Here's how the part is built. I have some questions about the finished solid (model axes, mm). A direction names the side the tool comes from. Round coordinates to 2 decimals unless told otherwise and drop trailing zeros. Order: outer loops, then holes, each group sorted by start corner. A loop starts at its lowest first (then second) coordinate and runs counter-clockwise, first axis right, second up.
```python
from build123d import *

# Parameters (mm, degrees)
RADYUS1_R             = 10
IZIM2_R               = 3.75
KES_EKSTR_ZYON1_DEPTH = 10
RADYUS2_R             = 10
IZIM3_R               = 3.5
KES_EKSTR_ZYON2_DEPTH = 100.511524539


with BuildPart() as part:
    # Çizim1 → Döndür1 (revolve)
    with BuildSketch(Plane.XY):
        Polygon((158.555065461, 64.488475461), (158.555065461, 62.488475461), (48.555065461, 62.488475461), (48.555065461, 23.488475461), (888.555065461, 23.488475461), (888.555065461, 62.488475461), (778.555065461, 62.488475461), (778.555065461, 64.488475461), (688.555065461, 64.488475461), (688.555065461, 83.488475461), (248.555065461, 83.488475461), (248.555065461, 64.488475461), align=None)
    revolve(axis=Axis((48.555065461, 23.488475461, 0), (1, 0, 0)))

    # Radyus1
    radyus1_edges = [part.edges().sort_by_distance(p)[0] for p in [
        (48.555065461, -15.511524539, 0),
    ]]
    fillet(radyus1_edges, radius=RADYUS1_R)

    # Çizim2 → Kes-Ekstrüzyon1 (cut)
    with BuildSketch(Plane.ZY.offset(-48.555065461)):
        with Locations((0, 23.488475461)):
            Circle(IZIM2_R)
    extrude(amount=-KES_EKSTR_ZYON1_DEPTH, mode=Mode.SUBTRACT)

    # Radyus2
    radyus2_edges = [part.edges().sort_by_distance(p)[0] for p in [
        (888.555065461, -15.511524539, 0),
    ]]
    fillet(radyus2_edges, radius=RADYUS2_R)

    # Çizim3 → Kes-Ekstrüzyon2 (cut, through all)
    with BuildSketch(Plane(origin=(0, 63, 0), x_dir=(1, 0, 0), z_dir=(0, 1, 0))):
        with Locations((63.555065461, 0)):
            Circle(IZIM3_R)
        with Locations((873.555065461, 0)):
            Circle(IZIM3_R)
    extrude(amount=-KES_EKSTR_ZYON2_DEPTH, mode=Mode.SUBTRACT)


solid = part.part
```
1) I'm going to push flat-ended pins straight in: pin 1 (3 mm diameter, centred on x = 761.5, z = -6.5, fed in from -Y); pin 2 (10 mm diameter, centred on y = 52.5, z = 36.5, fed in from -X); pin 3 (10 mm diameter, centred on x = 472.5, y = 26, fed in from -Z); pin 4 (6.5 mm diameter, centred on x = 873.56, z = 0, fed in from +Y). Where does each tip first touch, or does it pass through?
2) If we section it at A-A (x = 364): Write out the boundary of the cut face in (y, z), plus the area to 3 significant figures.
3) If we section it at D-D (x = 120): Write out the boundary of the cut face in (y, z), plus the area to 3 significant figures.
4) If we section it at B-B (y = 8.5): Give the number of separate pieces and of enclosed holes in the cut face, plus the area to 3 significant figures.
5) For faces 1 (the cylindrical face through (465.475, -36.454, 2.638)), 2 (the cylindrical face through (107.86, 60.69, 11.71)), 3 (the flat face through (688.555, -16, -12)), which set-ups out of +Z, -Z, +X, -X, +Y, -Y let a thin tool reach every point of the face, with its end or its side?
6) If we section it at C-C (y = 74): Write out the boundary of the cut face in (x, z), plus the area to 3 significant figures.
7) I need wall thicknesses on line 1 (X direction, y = 17, z = 0); line 2 (X direction, y = 24.5, z = 0); line 3 (X direction, y = 43.5, z = -53). Which ranges of each line are inside material? Lowest first, please.
Solutions:
1. pin 1: stops at y = -17.21
1. pin 2: stops at x = 248.56
1. pin 3: stops at z = -60
1. pin 4: passes through
2. outline: circle Ø120 at (23.49, 0)
2. area: 11,300 mm2
3. outline: circle Ø78 at (23.49, 0)
3. area: 4,780 mm2
4. separate pieces: 1
4. enclosed holes: 2
4. area: 80,500 mm2
5. face 1: +X, -X
5. face 2: -X
5. face 3: +X
6. outline: (248.56, -32.38) - (688.56, -32.38) - (688.56, 32.38) - (248.56, 32.38) - close
6. area: 28,500 mm2
7. line 1: x = 48.56 to 60.06, 67.06 to 870.06, 877.06 to 888.56
7. line 2: x = 58.56 to 60.06, 67.06 to 870.06, 877.06 to 888.56
7. line 3: x = 248.56 to 688.56
